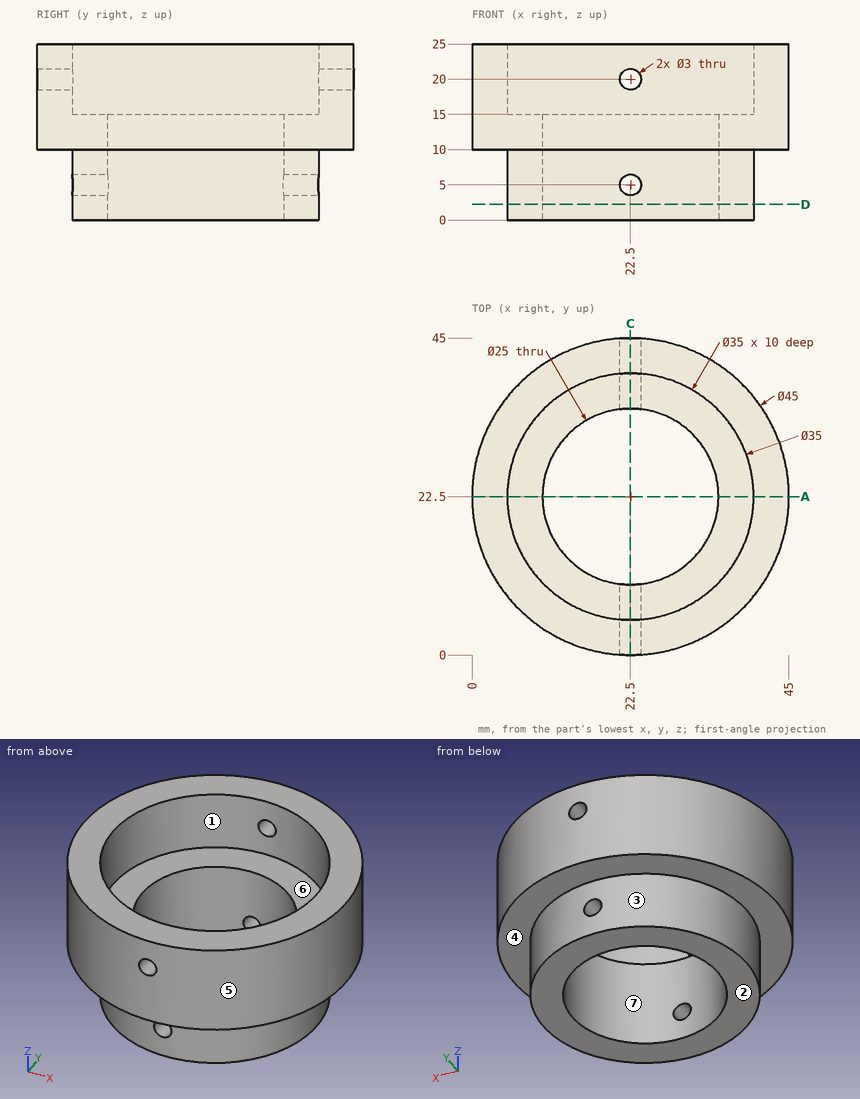
Design review of the part shown in the three views and the two pictorial views. Dimensions are in mm from the part's minimum x, y and z. A direction names the side the tool comes from. Give positions to 0.01 mm unless a question says otherwise; leave off trailing zeros. Loops run counter-clockwise (first coordinate to the right, second up) from the corner with the lowest first, then second, coordinate; pieces in that order, holes last. Notation, with made-up numbers: (61.5, 31) -> (115.5, 31) arc R32 ccw to (115.5, 59) -> close; hole circle Ø10 at (53.25, -17.5). An arc over 180 degrees is marked (long way). Answer as a JSON object with one key per item and string values. Group by question number.
Q1. Take a section at C-C (x = 22.5). State how many separate pieces and enclosed holes the cut face has, plus the area to 3 significant figures.
Q2. Take a section at A-A (y = 22.5). Write out the cut boundary in (x, z).
Q3. Take a section at D-D (z = 2.25). Write out the cut boundary in (x, y), plus the area to 3 significant figures.
Q4. Wall thickness on line 1 along Z through (x, y) = (22.5, 39.5); line 2 along Y through (x, z) = (22.5, 17.75); line 3 along Z through (x, y) = (16.5, 40.5): over which ranges is each line inside the solid? List them lowest first.
Q5. Tool access review of the marked faces 1, 2 and 3: name each direction out of +Z, -Z, +X, -X, +Y, -Y from which nothing blocks a thin tool from reaching the whole face with its end or side.
Q6. Insertion check: pin 1 (1 mm diameter, centred on x = 33, z = 17.5, fed in from +Y); pin 2 (2 mm diameter, centred on x = 39, z = 10.5, fed in from +Y); pin 3 (10 mm diameter, centred on y = 12.5, z = 19, fed in from +X); pin 4 (10 mm diameter, centred on y = 26, z = 13, fed in from -X). Each pin has a flat end and moves straight along its axis. Give the tip position at first contact, or say it passes through.
Q7. Draft analysis for pull direction Y (two halves, no side actions). For the marked faces 4, 5, 6 and 7, state which applies: pulls with the +Y half, pulls with the -Y half, needs draft (parallel to the pull), parting line crosses it, or undercut.
Answer below:
{
 "1": {"separate pieces": "6", "enclosed holes": "0", "area": "240 mm2"},
 "2": {"outline": "(0, 10) -> (5, 10) -> (5, 0) -> (10, 0) -> (10, 15) -> (5, 15) -> (5, 25) -> (0, 25) -> close; (35, 0) -> (40, 0) -> (40, 10) -> (45, 10) -> (45, 25) -> (40, 25) -> (40, 15) -> (35, 15) -> close"},
 "3": {"outline": "circle Ø35 at (22.5, 22.5); hole circle Ø25 at (22.5, 22.5)", "area": "471 mm2"},
 "4": {"line 1": "z = 0 to 3.5, 6.5 to 15", "line 2": "y = 0 to 5, 40 to 45", "line 3": "z = 10 to 25"},
 "5": {"face 1": "+Z", "face 2": "-Z, +X, -X, +Y, -Y", "face 3": "-Z"},
 "6": {"pin 1": "stops at y = 42.66", "pin 2": "stops at y = 38.81", "pin 3": "stops at x = 44.44", "pin 4": "stops at x = 0"},
 "7": {"face 4": "needs draft", "face 5": "parting line crosses it", "face 6": "undercut", "face 7": "undercut"}
}
